Check sheet for the modelled part. Datum: model origin and axes. Units: mm. Face numbers are marked on the shaded views. Give positions to 0.01 mm unless a question says otherwise; leave off trailing zeros. Loops run counter-clockwise (first coordinate to the right, second up) from the corner with the lowest first, then second, coordinate; pieces in that order, holes last. Notation, with made-up numbers: M 12,59 L 28,59 A23 cw 28,88 Z; hole C 37,60.5 d2. An arc over 180 degrees is marked long. Put each result on its own line as item: value. Start each with the question number.
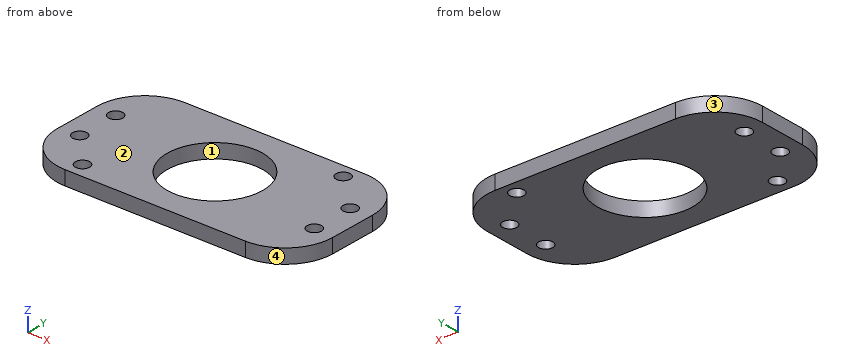
```python
from build123d import *

# Parameters (mm, degrees)
SKETCH1_W           = 58
SKETCH1_H           = 30
BOSS_EXTRUDE1_DEPTH = 3
FILLET1_R           = 10
SKETCH2_R           = 1.5
CUT_EXTRUDE1_DEPTH  = 3
SKETCH3_R           = 1.5
CUT_EXTRUDE2_DEPTH  = 3
SKETCH4_R           = 10
CUT_EXTRUDE3_DEPTH  = 10


with BuildPart() as part:
    # Sketch1 → Boss-Extrude1 (new body)
    with BuildSketch(Plane.XY):
        with Locations((-7.345808821, 32.102080843)):
            Rectangle(SKETCH1_W, SKETCH1_H)
    extrude(amount=BOSS_EXTRUDE1_DEPTH)

    # Fillet1
    fillet1_edges = [part.edges().sort_by_distance(p)[0] for p in [
        (21.654191179, 17.102080843, 1.5),
        (-36.345808821, 17.102080843, 1.5),
        (-36.345808821, 47.102080843, 1.5),
        (21.654191179, 47.102080843, 1.5),
    ]]
    fillet(fillet1_edges, radius=FILLET1_R)

    # Sketch2 → Cut-Extrude1 (cut)
    with BuildSketch(Plane.XY.offset(3)):
        with Locations((17.369191179, 27.602080843)):
            Circle(SKETCH2_R)
        with Locations((17.369191179, 36.602080843)):
            Circle(SKETCH2_R)
    cut_extrude1 = extrude(amount=-CUT_EXTRUDE1_DEPTH, mode=Mode.SUBTRACT)

    # Mirror1: Cut-Extrude1 across plane
    add(cut_extrude1.mirror(Plane(origin=(-7.345808821, 0, 0), x_dir=(0, 0, 1), z_dir=(1, 0, 0))), mode=Mode.SUBTRACT)

    # Sketch3 → Cut-Extrude2 (cut)
    with BuildSketch(Plane.XY.offset(3)):
        with Locations((-25.326377841, 20.27169556)):
            Circle(SKETCH3_R)
        with Locations((9.503472923, 44.194442915)):
            Circle(SKETCH3_R)
    extrude(amount=-CUT_EXTRUDE2_DEPTH, mode=Mode.SUBTRACT)

    # Sketch4 → Cut-Extrude3 (cut)
    with BuildSketch(Plane.XY.offset(3)):
        with Locations((-7.345808821, 32.102080843)):
            Circle(SKETCH4_R)
    extrude(amount=-CUT_EXTRUDE3_DEPTH, mode=Mode.SUBTRACT)


solid = part.part
```
Q1. Depth check by flat-ended pin: P1, Ø2.5, axis at x = 17.37, y = 27.6, coming from the -Z side; P2, Ø3.5, axis at x = -25.33, y = 20.27, coming from the -Z side. Enter the tip coordinate at first touch or a pass-through.
Q2. Section check A-A, the plane y = 40.25. Record the cut outline in (x, z).
Q3. Thickness scan on line 1 along X through (y, z) = (34.75, 0.7); line 2 along Y through (x, z) = (17.5, 1.2); line 3 along Y through (x, z) = (-9.5, 1). Record the ranges inside material, lowest first. Write a range as [from, to].
Q4. Mould release check, pull along Y, two halves, no side actions. Record for the marked faces 1, 2, 3 and 4: pulls with the +Y half, pulls with the -Y half, needs draft (parallel to the pull), parting line crosses it, or undercut.
Q5. Section check B-B, the plane x = -12. Record the cut outline in (y, z).
Q6. Section check C-C, the plane z = 0.7. Record the cut outline in (x, y).
Found:
1. P1: passes through
1. P2: stops at z = 0
2. outline: M -35.84,0 L -13.14,0 L -13.14,3 L -35.84,3 Z; M -1.55,0 L 21.15,0 L 21.15,3 L -1.55,3 Z
3. line 1: x = [-36.35, -16.99], [2.3, 21.65]
3. line 2: y = [18.99, 26.11], [29.1, 35.11], [38.1, 45.22]
3. line 3: y = [17.1, 22.34], [41.87, 47.1]
4. face 1: undercut
4. face 2: needs draft
4. face 3: pulls with the +Y half
4. face 4: pulls with the -Y half
5. outline: M 17.1,0 L 23.25,0 L 23.25,3 L 17.1,3 Z; M 40.95,0 L 47.1,0 L 47.1,3 L 40.95,3 Z
6. outline: M -36.35,27.1 A10 ccw -26.35,17.1 L 11.65,17.1 A10 ccw 21.65,27.1 L 21.65,37.1 A10 ccw 11.65,47.1 L -26.35,47.1 A10 ccw -36.35,37.1 Z; hole C -32.06,27.6 d3; hole C -32.06,36.6 d3; hole C -25.33,20.27 d3; hole C -7.35,32.1 d20; hole C 9.5,44.19 d3; hole C 17.37,27.6 d3; hole C 17.37,36.6 d3
